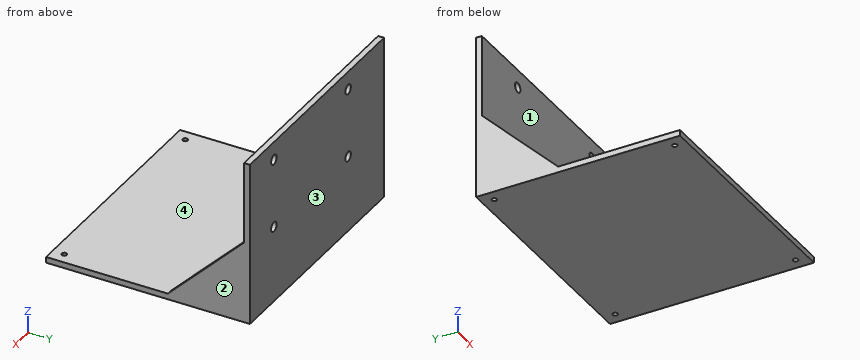
from build123d import *

# Parameters (mm, degrees)
F1_DEPTH  = 406
F2_W      = 10
F2_H      = 130
F3_DEPTH  = 130
F6_DEPTH  = 406.001
F7_R      = 8.25
F8_DEPTH  = 348.001
F9_R      = 4.25
F10_DEPTH = 280.001


with BuildPart() as f1:
    # F0 (on Right) → F1 (new body)
    with BuildSketch(Plane.YZ):
        Polygon((10, 135), (0, 135), (0, -135), (-338, -135), (-338, -145), (10, -145), align=None)
    extrude(amount=F1_DEPTH)

    # F2 (on face) → F3 (join)
    with BuildSketch(Plane.XZ):
        with Locations((5, -70)):
            Rectangle(F2_W, F2_H)
        with Locations((401, -70)):
            Rectangle(F2_W, F2_H)
    extrude(amount=F3_DEPTH)

    # F5 (on face) + F4 (on face) → F6 (cut, through all)
    with BuildSketch(Plane(origin=(0, 0, 0), x_dir=(0, -1, 0), z_dir=(-1, 0, 0))):
        Polygon((130, -5), (0, -5), (130, -135), align=None)
    with BuildSketch(Plane.YZ.offset(406)):
        Polygon((-130, -135), (0, -5), (-130, -5), align=None)
    extrude(amount=-F6_DEPTH, mode=Mode.SUBTRACT)

    # F7 (on face) → F8 (cut, through all)
    with BuildSketch(Plane(origin=(0, 10, 0), x_dir=(-1, 0, 0), z_dir=(0, 1, 0))):
        with Locations((-333.5, 104)):
            Circle(F7_R)
        with Locations((-333.5, -14)):
            Circle(F7_R)
        with Locations((-108.5, -14)):
            Circle(F7_R)
        with Locations((-108.5, 104)):
            Circle(F7_R)
    extrude(amount=-F8_DEPTH, mode=Mode.SUBTRACT)

    # F9 (on face) → F10 (cut, through all)
    with BuildSketch(Plane(origin=(0, 0, -145), x_dir=(1, 0, 0), z_dir=(0, 0, -1))):
        with Locations((20, 318)):
            Circle(F9_R)
        with Locations((386, 318)):
            Circle(F9_R)
        with Locations((20, 10)):
            Circle(F9_R)
        with Locations((386, 10)):
            Circle(F9_R)
    extrude(amount=-F10_DEPTH, mode=Mode.SUBTRACT)


solid = f1.part
Can you work these out from the model? Positions are in its coordinate system, mm. Face numbers are marked on the shaded views. Coordinates: 2 decimals unless noted, no trailing zeros. Write each loop counter-clockwise with the first axis right and the second up, starting at its lowest first coordinate (ties: lowest second). Pieces come first, ordered by that corner, then holes. Notation, with made-up numbers: (-10.5, -38) -> (-4.5, -38) arc R15 ccw to (-4.5, -15) -> close; hole circle Ø4 at (64.5, 25). An arc over 180 degrees is marked (long way). Answer as CSV lines item,"result".
1) If I drill on line 1 (Z direction, x = 333, y = 3); line 2 (X direction, y = -10, z = -138.5); line 3 (Y direction, x = 386, z = -142), over which ranges is the centre line in solid material (lowest first)? Write a range as from..to.
Check result:
line 1,"-145..-22.23, -5.77..95.77, 112.23..135"
line 2,"0..15.75, 24.25..381.75, 390.25..406"
line 3,"-338..-322.25, -313.75..-14.25, -5.75..10"
2) If we section it at B-B on y = -56.5: Please give me the cut outline in (x, z).
Check result:
outline,"(0, -145) -> (406, -145) -> (406, -61.5) -> (396, -61.5) -> (396, -135) -> (10, -135) -> (10, -61.5) -> (0, -61.5) -> close"
3) If we mould it in two halves opening along X, with no side actions, what happens to the marked faces 1, 2, 3 and 4? For each: +X half, -X half, draft (parallel to the pull), parting line (faces both ways), or undercut.
Check result:
face 1,"undercut"
face 2,"+X half"
face 3,"draft"
face 4,"undercut"
4) If we section it at D-D on x = 217: Please give me the cut outline in (y, z).
Check result:
outline,"(-338, -145) -> (10, -145) -> (10, 135) -> (0, 135) -> (0, -135) -> (-338, -135) -> close"
5) If we section it at A-A on z = -14: Please give me the cut outline in (x, y), then the cut area to 3 significant figures.
Check result:
outline,"(0, -9) -> (10, -9) -> (10, 0) -> (100.25, 0) -> (100.25, 10) -> (0, 10) -> close; (116.75, 0) -> (325.25, 0) -> (325.25, 10) -> (116.75, 10) -> close; (341.75, 0) -> (396, 0) -> (396, -9) -> (406, -9) -> (406, 10) -> (341.75, 10) -> close"
area,"3,910 mm²"
6) If we section it at C-C on z = -82: Please give me the cut outline in (x, y), then the cut area to 3 significant figures.
Check result:
outline,"(0, -77) -> (10, -77) -> (10, 0) -> (396, 0) -> (396, -77) -> (406, -77) -> (406, 10) -> (0, 10) -> close"
area,"5,600 mm²"
7) Will these pins go through, and if not, where does the flat tip stop? P1, Ø10, axis at x = 153.5, z = 4, coming from the -Y side; P2, Ø13.5, axis at x = 386, y = -318, coming from the +Z side; P3, Ø5, axis at x = 386, y = -10, coming from the +Z side; P4, Ø21.5, axis at x = 108.5, z = 104, coming from the +Y side.
Check result:
P1,"y = 0"
P2,"z = -135"
P3,"through"
P4,"y = 10"
